Autodesk Inventor part; units mm, degrees
ref_plane "YZ Plane" through (0, 0, 0) normal (1, 0, 0) x (0, 1, 0)
ref_plane "XZ Plane" through (0, 0, 0) normal (0, 1, 0) x (-1, 0, 0)
ref_plane "XY Plane" through (0, 0, 0) normal (0, 0, 1) x (1, 0, 0)
sketch "スケッチ1" plane through (0, 0, 0) normal (0, 0, 1) x (1, 0, 0)
  line L0 (0, 0) -> (17.8, 0)
  line L1 (17.8, 0) -> (17.8, 6.4)
  line L2 (17.8, 6.4) -> (28, 6.4)
  line L3 (28, 6.4) -> (28, 41.8)
  line L4 (28, 41.8) -> (-10.2, 41.8)
  line L5 (-10.2, 41.8) -> (-10.2, 6.4)
  line L6 (-10.2, 6.4) -> (0, 6.4)
  line L7 (0, 6.4) -> (0, 0)
  line L8 (0, 2.7) -> (17.8, 2.7) construction
  circle A0 centre (5.7, 2.7) radius 1.7
  circle A1 centre (12.1, 2.7) radius 1.7
  circle A2 centre (23.1, 10.1) radius 1.7
  dimension "d0" = 3.4
  dimension "d1" = 17.8
  dimension "d2" = 6.4
  dimension "d3" = 5.7
  dimension "d4" = 2.7
  dimension "d5" = 6.4
  dimension "d6" = 35.4
  dimension "d7" = 38.2
  dimension "d8" = 10.2
  dimension "d9" = 4.9
  dimension "d10" = 3.7
extrude "押し出し1" add sketch "スケッチ1" along normal blind 1.5
chamfer "面取り1" distance 2 angle 45 2 edges at (17.8, 6.4, 0.75) (0, 6.4, 0.75)
properties part number "pixy"
The listing builds one solid part. Answer for the finished solid, in the listing's coordinates (mm). A direction names the side the tool comes from. Coordinates: 2 decimals unless noted, no trailing zeros. Write each loop counter-clockwise with the first axis right and the second up, starting at its lowest first coordinate (ties: lowest second). Pieces come first, ordered by that corner, then holes. Notation, with made-up numbers: (31, 65.25) - (80, 65.25) arc R22 ccw to (80, 75.25) - close; hole circle Ø8 at (78, -25.5). An arc over 180 degrees is marked (long way). Return JSON: item names as keys, results as strings.
1. The part is cut by section D-D on y = 10.1. Determine the outline of the cut face in (x, z), then the cut area to 3 significant figures.
Final values:
{"outline": "(-10.2, 0) - (21.4, 0) - (21.4, 1.5) - (-10.2, 1.5) - close; (24.8, 0) - (28, 0) - (28, 1.5) - (24.8, 1.5) - close", "area": "52.2 mm^2"}
2. Which of the six approach directions +Z, -Z, +X, -X, +Y, -Y give full straight-line access (tool end or side, diameter ignored) to faces 1 (the face through (0, 2, 1)), 2 (the face through (13.67, 3.35, 0.74)), 3 (the face through (17.8, 2, 1))?
Final values:
{"face 1": "+Z, -Z, -X, -Y", "face 2": "+Z, -Z", "face 3": "+Z, -Z, +X, -Y"}
3. The part is cut by section B-B on x = 23.1. Determine the outline of the cut face in (y, z).
Final values:
{"outline": "(6.4, 0) - (8.4, 0) - (8.4, 1.5) - (6.4, 1.5) - close; (11.8, 0) - (41.8, 0) - (41.8, 1.5) - (11.8, 1.5) - close"}
4. Consider line 1 along Y through (x, z) = (23.1, 0.6); line 2 along Y through (x, z) = (5.7, 0.75); line 3 along Y through (x, z) = (-3, 0.75). Determine where each line is inside the solid, lowest interval first.
Final values:
{"line 1": "6.4 to 8.4, 11.8 to 41.8", "line 2": "0 to 1, 4.4 to 41.8", "line 3": "6.4 to 41.8"}
5. The part is cut by section C-C on z = 0.45. Determine the outline of the cut face in (x, y).
Final values:
{"outline": "(-10.2, 6.4) - (-2, 6.4) - (0, 4.4) - (0, 0) - (17.8, 0) - (17.8, 4.4) - (19.8, 6.4) - (28, 6.4) - (28, 41.8) - (-10.2, 41.8) - close; hole circle Ø3.4 at (5.7, 2.7); hole circle Ø3.4 at (12.1, 2.7); hole circle Ø3.4 at (23.1, 10.1)"}
6. For a pull along X with two mould halves and no side action, classify faces 4 (the face through (9, 21, 1.5)), 5 (the face through (21.4, 10.03, 0.74)), 6 (the face through (-1, 5.4, 0.8)) as +X half, -X half, draft (parallel to the pull), parting line (faces both ways), or undercut.
Final values:
{"face 4": "draft", "face 5": "undercut", "face 6": "-X half"}
7. The part is cut by section A-A on y = 2.7. Determine the outline of the cut face in (x, z), then the cut area to 3 significant figures.
Final values:
{"outline": "(0, 0) - (4, 0) - (4, 1.5) - (0, 1.5) - close; (7.4, 0) - (10.4, 0) - (10.4, 1.5) - (7.4, 1.5) - close; (13.8, 0) - (17.8, 0) - (17.8, 1.5) - (13.8, 1.5) - close", "area": "16.5 mm^2"}
